Geometry check sheet. Reference: drawing and pictorial views, mm from the part's lowest x, y, z. Give positions to 0.01 mm unless a question says otherwise; leave off trailing zeros. Loops run counter-clockwise (first coordinate to the right, second up) from the corner with the lowest first, then second, coordinate; pieces in that order, holes last. Notation, with made-up numbers: (-37.5, 43) - (18.5, 43) arc R18 ccw to (18.5, 63) - close; hole circle Ø4 at (-29.5, -14.75). An arc over 180 degrees is marked (long way). Use CSV: the item, a comma, the result in double quotes.
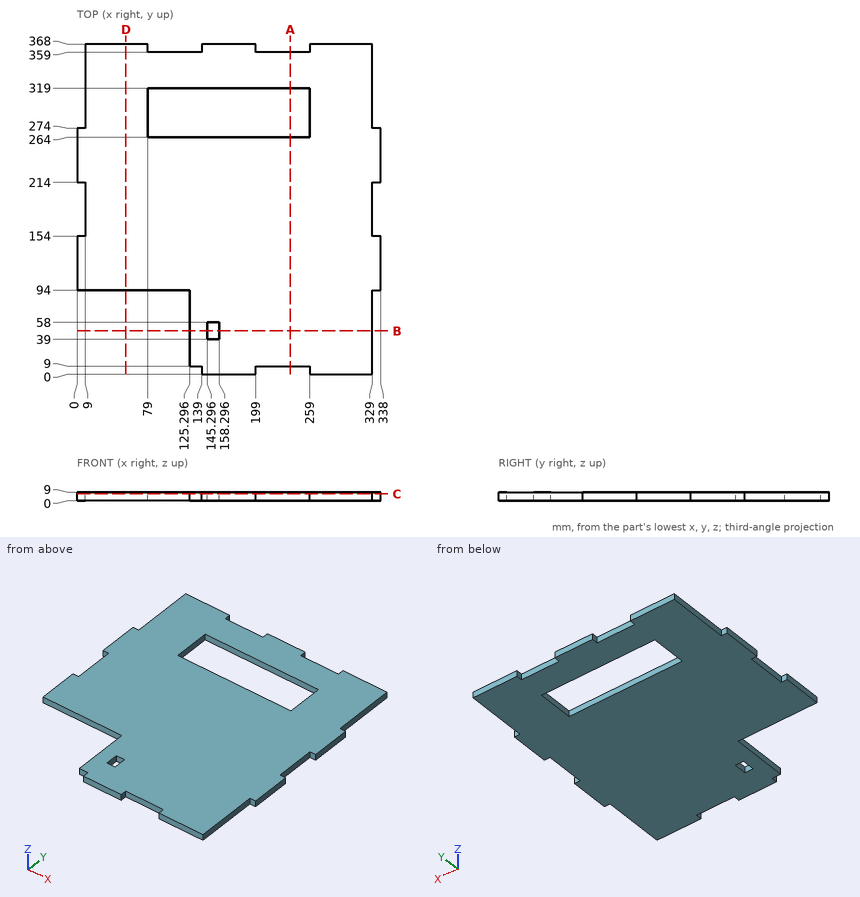
1. Sectioned sample at D-D, the plane x = 54.5. Record the boundary of the cut face in (y, z), and give its area (3 significant figures).
Completed:
outline,"(94, 0) - (368, 0) - (368, 9) - (94, 9) - close"
area,"2,470 mm²"
2. Go/stop test with flat-tipped pins: pin 1 Ø1 at (x, z) = (227, 8) entering from -Y; pin 2 Ø4.5 at (x, z) = (333, 4.5) entering from -Y; pin 3 Ø4.5 at (y, z) = (300, 4) entering from -X. Record where each tip stops, or that it passes through.
Completed:
pin 1,"stops at y = 9"
pin 2,"stops at y = 94"
pin 3,"stops at x = 9"
3. Sectioned sample at B-B, the plane y = 48.5. Record the boundary of the cut face in (x, z).
Completed:
outline,"(125.3, 0) - (145.3, 0) - (145.3, 9) - (125.3, 9) - close; (158.3, 0) - (329, 0) - (329, 9) - (158.3, 9) - close"
4. Scan lines: line 1 along Y through (x, z) = (90.5, 4.75); line 2 along X through (y, z) = (313, 4.5); line 3 along Y through (x, z) = (247, 3.75). Record each from-to range of solid material in increasing order.
Completed:
line 1,"y = 94 to 264, 319 to 359"
line 2,"x = 9 to 79, 259 to 329"
line 3,"y = 9 to 264, 319 to 359"
5. Sectioned sample at A-A, the plane x = 237.5. Record the boundary of the cut face in (y, z).
Completed:
outline,"(9, 0) - (264, 0) - (264, 9) - (9, 9) - close; (319, 0) - (359, 0) - (359, 9) - (319, 9) - close"
6. Sectioned sample at C-C, the plane z = 7.5. State how many separate pieces and enclosed holes the cut face has, and give its area (3 significant figures).
Completed:
separate pieces,"1"
enclosed holes,"2"
area,"97,100 mm²"
